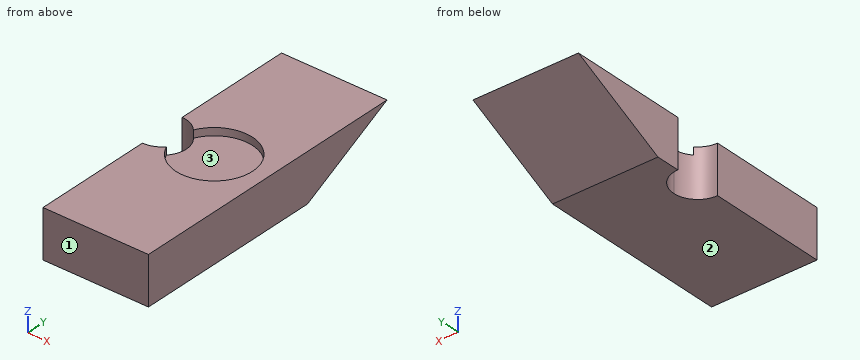
```python
from build123d import *

# Parameters (mm, degrees)
F1_DEPTH = 27.94
F2_R     = 10.16
F3_DEPTH = 2
F5_DEPTH = 25.4


with BuildPart() as f1:
    # F0 (on Right) → F1 (new body)
    with BuildSketch(Plane.YZ):
        Polygon((0, 12.7), (0, 0), (50.8, 0), (76.2, 12.7), align=None)
    extrude(amount=F1_DEPTH)

    # F2 (on face) → F3 (cut)
    with BuildSketch(Plane.XY.offset(12.7)):
        with Locations((13.97, 37.846)):
            Circle(F2_R)
    extrude(amount=-F3_DEPTH, mode=Mode.SUBTRACT)

    # F4 (on Top) → F5 (cut)
    with BuildSketch(Plane.XY):
        with BuildLine():
            ThreePointArc((0, 44.45), (-6.35, 38.1), (0, 31.75))
            Line((0, 31.75), (0, 38.1))
            Line((0, 38.1), (0, 44.45))
        make_face()
        with BuildLine():
            Line((0, 38.1), (0, 31.75))
            ThreePointArc((0, 31.75), (4.490128, 33.609872), (6.35, 38.1))
            Line((6.35, 38.1), (0, 38.1))
        make_face()
        with BuildLine():
            Line((0, 44.45), (0, 38.1))
            Line((0, 38.1), (6.35, 38.1))
            ThreePointArc((6.35, 38.1), (4.490128, 42.590128), (0, 44.45))
        make_face()
    extrude(amount=F5_DEPTH, mode=Mode.SUBTRACT)


solid = f1.part
```
Check sheet for the modelled part. Datum: model origin and axes. Units: mm. Face numbers are marked on the shaded views. Round coordinates to 2 decimals unless told otherwise and drop trailing zeros. Order: outer loops, then holes, each group sorted by start corner. A loop starts at its lowest first (then second) coordinate and runs counter-clockwise, first axis right, second up. Notation, with made-up numbers: M -34.75,-9 L -2.75,-9 A21 ccw -2.75,27 Z; hole C -5.75,70.25 d9. An arc over 180 degrees is marked long. Answer in a Markdown table with one row per item.
(1) Section check B-B on x = 13.97. Record the boundary of the cut face in (y, z), plus the area to 3 significant figures.
Findings:
| item | result |
|---|---|
| outline | M 0,0 L 50.8,0 L 76.2,12.7 L 48.01,12.7 L 48.01,10.7 L 27.69,10.7 L 27.69,12.7 L 0,12.7 Z |
| area | 766 mm^2 |
(2) Draft check along Y on the marked faces 1, 2 and 3. Enter one of: +Y half, -Y half, draft (parallel to the pull), parting line (faces both ways), or undercut.
Findings:
| item | result |
|---|---|
| face 1 | -Y half |
| face 2 | draft |
| face 3 | undercut |
(3) Section check A-A on z = 5.5. Record the boundary of the cut face in (x, y), plus the area to 3 significant figures.
Findings:
| item | result |
|---|---|
| outline | M 0,0 L 27.94,0 L 27.94,61.8 L 0,61.8 L 0,44.45 A6.35 cw 0,31.75 Z |
| area | 1,660 mm^2 |
(4) Section check C-C on y = 29. Record the boundary of the cut face in (x, z).
Findings:
| item | result |
|---|---|
| outline | M 0,0 L 27.94,0 L 27.94,12.7 L 18.97,12.7 L 18.97,10.7 L 8.97,10.7 L 8.97,12.7 L 0,12.7 Z |
(5) Material ranges on line 1 along Y through (x, z) = (13.97, 11.1); line 2 along Y through (x, z) = (13.97, 11.4); line 3 along Z through (x, y) = (6, 41), recorded low to high. Write a range as from..to.
Findings:
| item | result |
|---|---|
| line 1 | y = 0..27.69, 48.01..73 |
| line 2 | y = 0..27.69, 48.01..73.6 |
| line 3 | z = 0..10.7 |
(6) Gauge pin test, flat ends, axial feed: pin 1 (5 mm diameter, centred on y = 64, z = 5, fed in from +X); pin 2 (5 mm diameter, centred on x = 22, z = 5.5, fed in from +Y). Record the tip position at first contact, or that the pin passes through.
Findings:
| item | result |
|---|---|
| pin 1 | stops at x = 27.94 |
| pin 2 | stops at y = 66.8 |
(7) Section check D-D on z = 2.25. Record the boundary of the cut face in (x, y), plus the area to 3 significant figures.
Findings:
| item | result |
|---|---|
| outline | M 0,0 L 27.94,0 L 27.94,55.3 L 0,55.3 L 0,44.45 A6.35 cw 0,31.75 Z |
| area | 1,480 mm^2 |
